Source: CAD feature listing. Evaluate the final solid. Frame: model axes, mm. Face numbers are marked on the shaded views. A direction names the side the tool comes from. Round coordinates to 2 decimals unless told otherwise and drop trailing zeros. Order: outer loops, then holes, each group sorted by start corner. A loop starts at its lowest first (then second) coordinate and runs counter-clockwise, first axis right, second up. Notation, with made-up numbers: (8.5, -31) - (34.5, -31) arc R9 ccw to (34.5, -19) - close; hole circle Ø9 at (-7, 86.5). An arc over 180 degrees is marked (long way). Return JSON: item names as keys, results as strings. Group by question number.
1) Section B-B, the plane z = -105. Return loops of the section in (x, y), plus the area to 3 significant figures.
2) Contact query for flat-ended pins moving along their axis: P1, Ø6, axis at y = -123, z = -128.5, coming from the +X side; P2, Ø2, axis at y = -237.5, z = -168, coming from the -X side; P3, Ø11, axis at y = -105, z = -124, coming from the -X side. Output: stop coordinate, or through.
3) Mould query, pull axis X, two halves, no side actions, for the marked faces 1, 2 and 3. Classes: pulls with the +X half, pulls with the -X half, needs draft (parallel to the pull), parting line crosses it, or undercut.
4) Access query for the marked faces 4, 5 and 6. Directions: +Z, -Z, +X, -X, +Y, -Y. A direction counts if a zero-diameter tool reaches every point of the face in a straight line with its end or side. Return the directions, or none.
5) Section C-C, the plane x = -68. Return loops of the section in (y, z).
6) Section D-D, the plane x = 41. Return loops of the section in (y, z), plus the area to 3 significant figures.
7) Section A-A, the plane z = -130. Return loops of the section in (x, y), plus the area to 3 significant figures.
8) Ray query, line 1 (Y direction, x = 0, z = -183) (3 decimals); line 2 (X direction, y = -232, z = -181.75) (3 decimals); line 3 (X direction, y = -160.5, z = -160.5). Return the intervals inside material, ascending. Write a range as from..to.
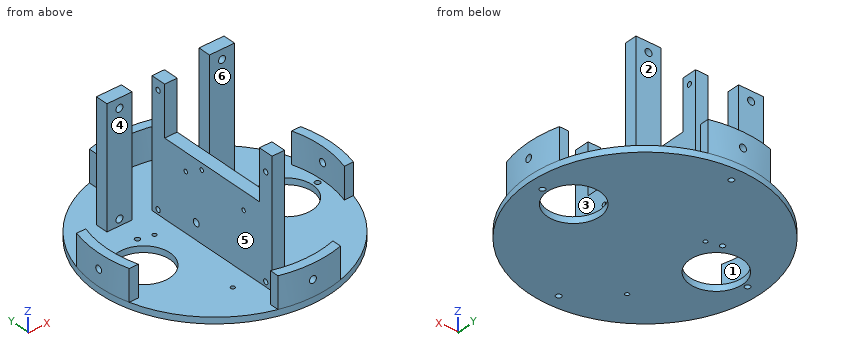
```python
from build123d import *

# Parameters (mm, degrees)
CYLINDER135_R     = 2.8
CYLINDER135_DEPTH = 300
CYLINDER136_R     = 2.8
CYLINDER136_DEPTH = 300
SKETCH043_R       = 2.125
EXTRUDE025_DEPTH  = 20
EXTRUDE021_DEPTH  = 30
SKETCH034_W       = 20
SKETCH034_H       = 95
SKETCH034_R       = 2.8
EXTRUDE016_DEPTH  = 10
SKETCH035_R       = 2
SKETCH035_R_2     = 1.625
EXTRUDE017_DEPTH  = 10
SKETCH033_R       = 93
SKETCH033_R_2     = 21
SKETCH033_R_3     = 2
SKETCH033_R_4     = 1.625
EXTRUDE015_DEPTH  = 5


with BuildPart() as cylinder135:
    # Cylinder135 → Cylinder135 (new body)
    with BuildSketch(Plane(origin=(0, 0, 90), x_dir=(1, 0, 0), z_dir=(0, -1, 0))):
        Circle(CYLINDER135_R)
    extrude(amount=CYLINDER135_DEPTH)


with BuildPart() as m4heatsetcuts002:
    # Cylinder136 → Cylinder136 (new body)
    with BuildSketch(Plane(origin=(-150, -150, 90), x_dir=(0, 1, 0), z_dir=(1, 0, 0))):
        Circle(CYLINDER136_R)
    extrude(amount=CYLINDER136_DEPTH)

    # Fusion086: union Cylinder135
    add(cylinder135.part)


with BuildPart() as m4heatsetcuts002_1:
    # Fusion086 placement: moved
    add(m4heatsetcuts002.part.moved(Location((0, 0, -257))))


with BuildPart() as m4vercuts:
    # Sketch043 → Extrude025 (new body)
    with BuildSketch(Plane.XY):
        with Locations((0, -68)):
            Circle(SKETCH043_R)
        with Locations((82, -150)):
            Circle(SKETCH043_R)
        with Locations((0, -232)):
            Circle(SKETCH043_R)
        with Locations((-82, -150)):
            Circle(SKETCH043_R)
    extrude(amount=EXTRUDE025_DEPTH)


with BuildPart() as m4vercuts_1:
    # Extrude025 placement: moved
    add(m4vercuts.part.moved(Location((0, 0, -194.5))))


with BuildPart() as obj1:
    # Sketch039 → Extrude021 (new body)
    with BuildSketch(Plane.XY):
        with BuildLine():
            ThreePointArc((-89.576783, -125), (-93, -150), (-89.576783, -175))
            Line((-89.576783, -175), (-82.286086, -175))
            ThreePointArc((-82.286086, -125), (-86, -150), (-82.286086, -175))
            Line((-89.576783, -125), (-82.286086, -125))
        make_face()
        with BuildLine():
            ThreePointArc((25, -60.423217), (0, -57), (-25, -60.423217))
            Line((-25, -60.423217), (-25, -67.713914))
            ThreePointArc((25, -67.713914), (0, -64), (-25, -67.713914))
            Line((25, -60.423217), (25, -67.713914))
        make_face()
        with BuildLine():
            ThreePointArc((89.576783, -175), (93, -150), (89.576783, -125))
            Line((89.576783, -125), (82.286086, -125))
            ThreePointArc((82.286086, -175), (86, -150), (82.286086, -125))
            Line((89.576783, -175), (82.286086, -175))
        make_face()
        with BuildLine():
            ThreePointArc((-25, -239.576783), (0, -243), (25, -239.576783))
            Line((25, -239.576783), (25, -232.286086))
            ThreePointArc((-25, -232.286086), (0, -236), (25, -232.286086))
            Line((-25, -239.576783), (-25, -232.286086))
        make_face()
    extrude(amount=EXTRUDE021_DEPTH)


with BuildPart() as obj1_1:
    # Extrude021 placement: moved
    add(obj1.part.moved(Location((0, 0, -185))))


with BuildPart() as fanholder:
    # Sketch034 → Extrude016 (new body)
    with BuildSketch(Plane.XZ):
        with Locations((-41, -132.5)):
            Rectangle(SKETCH034_W, SKETCH034_H)
        with Locations((-41, -92.75)):
            Circle(SKETCH034_R, mode=Mode.SUBTRACT)
        with Locations((-41, -174.75)):
            Circle(SKETCH034_R, mode=Mode.SUBTRACT)
        with Locations((41, -132.5)):
            Rectangle(SKETCH034_W, SKETCH034_H)
        with Locations((41, -92.75)):
            Circle(SKETCH034_R, mode=Mode.SUBTRACT)
        with Locations((41, -174.75)):
            Circle(SKETCH034_R, mode=Mode.SUBTRACT)
    extrude(amount=EXTRUDE016_DEPTH)


with BuildPart() as fanholder_1:
    # Extrude016 placement: moved
    add(fanholder.part.moved(Location((0, -98, 0))))


with BuildPart() as obj2:
    # Sketch035 → Extrude017 (new body)
    with BuildSketch(Plane.YZ):
        Polygon((-222, -80), (-210, -80), (-210, -120), (-120, -120), (-120, -80), (-108, -80), (-108, -180), (-222, -180), align=None)
        with Locations((-216, -94.75)):
            Circle(SKETCH035_R, mode=Mode.SUBTRACT)
        with Locations((-113.8, -87.8)):
            Circle(SKETCH035_R, mode=Mode.SUBTRACT)
        with Locations((-113.8, -176.2)):
            Circle(SKETCH035_R, mode=Mode.SUBTRACT)
        with Locations((-216, -176.2)):
            Circle(SKETCH035_R, mode=Mode.SUBTRACT)
        with Locations((-155.2, -125.25)):
            Circle(SKETCH035_R_2, mode=Mode.SUBTRACT)
        with Locations((-140, -134.25)):
            Circle(SKETCH035_R_2, mode=Mode.SUBTRACT)
        with Locations((-195, -134.25)):
            Circle(SKETCH035_R_2, mode=Mode.SUBTRACT)
    extrude(amount=EXTRUDE017_DEPTH)


with BuildPart() as obj2_1:
    # Extrude017 placement: moved
    add(obj2.part.moved(Location((-15, 0, 0))))


with BuildPart() as level4s001:
    # Sketch033 → Extrude015 (new body)
    with BuildSketch(Plane.XY):
        with Locations((0, -150)):
            Circle(SKETCH033_R)
        with Locations((-57, -150)):
            Circle(SKETCH033_R_2, mode=Mode.SUBTRACT)
        with Locations((-41.75, -126)):
            Circle(SKETCH033_R_3, mode=Mode.SUBTRACT)
        with Locations((-30.75, -129.1)):
            Circle(SKETCH033_R_4, mode=Mode.SUBTRACT)
        with Locations((-30.75, -203.5)):
            Circle(SKETCH033_R_4, mode=Mode.SUBTRACT)
        with Locations((57, -150)):
            Circle(SKETCH033_R_2, mode=Mode.SUBTRACT)
    extrude(amount=EXTRUDE015_DEPTH)


with BuildPart() as level4s001_1:
    # Extrude015 placement: moved
    add(level4s001.part.moved(Location((0, 0, -185))))

    # Fusion077: union fanHolder, obj2
    add(fanholder_1.part)
    add(obj2_1.part)

    # Fusion081: union obj1
    add(obj1_1.part)

    # Cut037: cut m4VerCuts
    add(m4vercuts_1.part, mode=Mode.SUBTRACT)

    # Cut039: cut m4HeatSetCuts002
    add(m4heatsetcuts002_1.part, mode=Mode.SUBTRACT)


solid = level4s001_1.part
```
Geometry check:
{
 "1": {"outline": "(-51, -108) - (-31, -108) - (-31, -98) - (-51, -98) - close; (-15, -222) - (-5, -222) - (-5, -210) - (-15, -210) - close; (-15, -120) - (-5, -120) - (-5, -108) - (-15, -108) - close; (31, -108) - (51, -108) - (51, -98) - (31, -98) - close", "area": "640 mm2"},
 "2": {"P1": "x = -5", "P2": "x = -25", "P3": "x = -51"},
 "3": {"face 1": "undercut", "face 2": "needs draft", "face 3": "undercut"},
 "4": {"face 4": "+Z, -X, -Y", "face 5": "+Z", "face 6": "+Z, +X, -Y"},
 "5": {"outline": "(-213.44, -185) - (-167.89, -185) - (-167.89, -180) - (-213.44, -180) - close; (-132.11, -185) - (-86.56, -185) - (-86.56, -180) - (-132.11, -180) - close"},
 "6": {"outline": "(-233.47, -185) - (-163.6, -185) - (-163.6, -180) - (-233.47, -180) - close; (-136.4, -185) - (-66.53, -185) - (-66.53, -180) - (-98, -180) - (-98, -177.55) - (-108, -177.55) - (-108, -180) - (-136.4, -180) - close; (-108, -171.95) - (-98, -171.95) - (-98, -95.55) - (-108, -95.55) - close; (-108, -89.95) - (-98, -89.95) - (-98, -85) - (-108, -85) - close", "area": "1,540 mm2"},
 "7": {"outline": "(-51, -108) - (-31, -108) - (-31, -98) - (-51, -98) - close; (-15, -222) - (-5, -222) - (-5, -108) - (-15, -108) - close; (31, -108) - (51, -108) - (51, -98) - (31, -98) - close", "area": "1,540 mm2"},
 "8": {"line 1": "-243..-234.125, -229.875..-70.125, -65.875..-57", "line 2": "-43.875..-2.125, 2.125..43.875", "line 3": "-92.41..-85.36, -15..-5, 85.36..92.41"}
}
